Design review of the part built by this model. Coordinates are the model's own, in mm. A direction names the side the tool comes from. Give positions to 0.01 mm unless a question says otherwise; leave off trailing zeros. Order: outer loops, then holes, each group sorted by start corner. A loop starts at its lowest first (then second) coordinate and runs counter-clockwise, first axis right, second up. Notation, with made-up numbers: (-29, -17) -> (13, -17) arc R17 cw to (13, 16) -> close; hole circle Ø3 at (-19.75, -14). An arc over 180 degrees is marked (long way). One line per item, written item: value. Start each with the question number.
1) Wall thickness on line 1 along Z through (x, y) = (15.78, 1); line 2 along Z through (x, y) = (-15.78, 0.8); line 3 along X through (y, z) = (0.7, -8.3): over which ranges is each line inside the solid? List them lowest first. Write a range as from..to.
2) Consider section C-C (z = -8.9). State the section outline as (x, y) points (3 decimals), plus the area to 3 significant figures.
3) The part is to be moulded in two halves that separate along Z. For faces 1 (the face through (11.499, 4.958, -2.515)), 2 (the face through (6, 5, 9.4)), 3 (the face through (3.62, 12.1, -10)), say which applies: released by +Z, released by -Z, zero draft, split by the parting line, or undercut.
4) Tool access review of faces 4 (the face through (-12, 3, -4)), 5 (the face through (-20.276, 6.24, -0.694)), 6 (the face through (-0.115, 4.958, -2.499)), 7 (the face through (14.19, 0.66, 8.23)), 8 (the face through (6, 8.71, 3)): name each direction out of +Z, -Z, +X, -X, +Y, -Y from which nothing blocks a thin tool from reaching the whole face with its end or side.
5) Consider section D-D (y = 7.25). State the section outline as (x, z) points, plus the area to 3 significant figures.
6) For pin 1 (1 mm diameter, centred on x = 4, y = 6.5, fed in from +Z); pin 2 (2 mm diameter, centred on x = 4.5, y = 4, fed in from -Z); pin 3 (3 mm diameter, centred on x = -7.5, z = -4.5, fed in from +Y), all flat-tipped, find the tip position at first contact; note any pin that passes through.
7) Consider section A-A (y = 4). State the section outline as (x, z) points, plus the area to 3 significant figures.
8) Consider section B-B (x = 10). State the section outline as (y, z) points.
Autodesk Inventor part; units mm, degrees
ref_plane "YZ Plane" through (0, 0, 0) normal (1, 0, 0) x (0, 1, 0)
ref_plane "XZ Plane" through (0, 0, 0) normal (0, 1, 0) x (-1, 0, 0)
ref_plane "XY Plane" through (0, 0, 0) normal (0, 0, 1) x (1, 0, 0)
sketch "Sketch1" plane through (0, 0, 0) normal (0, 1, 0) x (-1, 0, 0)
  line L0 (21.5, -10.6) -> (-21.5, -10.6)
  line L1 (-21.5, -10.6) -> (-21.5, 10.6)
  line L2 (-21.5, 10.6) -> (21.5, 10.6)
  line L3 (21.5, 10.6) -> (21.5, -10.6)
  point P0 (0, 0)
  dimension "d0" = 43
  dimension "d1" = 21.2
  dimension "d2" = 10.6
  dimension "d3" = 21.5
extrude "Extrusion1" add sketch "Sketch1" along normal blind 1.31
sketch "Sketch2" plane through (0, 1.31, 0) normal (0, 1, 0) x (1, 0, 0)
  line L0 (-12, 10) -> (-1.85, 10)
  line L1 (-1.85, 10) -> (-1.85, -2.4)
  line L2 (-1.85, -2.4) -> (-12, -2.4)
  line L3 (-12, -2.4) -> (-12, 10)
  line L4 (-21.5, -10.6) -> (21.5, -10.6)
  line L5 (-21.5, 10.6) -> (-21.5, -10.6)
  point P0 (0, 0)
  dimension "d6" = 12.4
  dimension "d7" = 10.15
  dimension "d8" = 8.2
  dimension "d9" = 9.5
extrude "Extrusion2" add sketch "Sketch2" along normal blind 4
sketch "Sketch3" plane through (0, 1.31, 0) normal (0, 1, 0) x (1, 0, 0)
  line L0 (0.6, 2.8) -> (10.8, 2.8)
  line L1 (11.8, 1.8) -> (11.8, -8.4)
  line L2 (10.8, -9.4) -> (0.6, -9.4)
  line L3 (-0.4, -8.4) -> (-0.4, 1.8)
  line L4 (-21.5, -10.6) -> (21.5, -10.6)
  line L5 (21.5, -10.6) -> (21.5, 10.6)
  arc A0 (0.6, 2.8) -> (-0.4, 1.8) centre (0.6, 1.8) ccw
  arc A1 (11.8, 1.8) -> (10.8, 2.8) centre (10.8, 1.8) ccw
  arc A2 (10.8, -9.4) -> (11.8, -8.4) centre (10.8, -8.4) ccw
  arc A3 (-0.4, -8.4) -> (0.6, -9.4) centre (0.6, -8.4) ccw
  point P0 (0, 0)
  dimension "d12" = 12.2
  dimension "d13" = 12.2
  dimension "d14" = 1.2
  dimension "d15" = 9.7
  dimension "d16" = 1
extrude "Extrusion3" add sketch "Sketch3" along normal blind 7.4
sketch "Sketch4" plane through (0, 1.31, 0) normal (0, 1, 0) x (1, 0, 0)
  line L0 (2.66, 10.1) -> (12.13, 10.1)
  line L1 (12.13, 10.1) -> (12.13, 5.79)
  line L2 (12.13, 5.79) -> (2.66, 5.79)
  line L3 (2.66, 5.79) -> (2.66, 10.1)
  line L4 (21.5, -10.6) -> (21.5, 10.6)
  line L5 (21.5, 10.6) -> (-21.5, 10.6)
  point P0 (0, 0)
  dimension "d19" = 4.31
  dimension "d20" = 9.47
  dimension "d21" = 9.37
  dimension "d22" = 0.5
extrude "Extrusion4" add sketch "Sketch4" along normal blind 10
sketch "Sketch5" plane through (0, 11.31, 0) normal (0, 1, 0) x (1, 0, 0)
  circle A0 centre (3.86, 8.9) radius 1.125
  line L0 (12.13, 10.1) -> (2.66, 10.1)
  line L1 (2.66, 10.1) -> (2.66, 5.79)
  point P0 (0, 0)
  point P1 (2.66, 9.2358)
  point P2 (2.66, 8.7642)
  point P3 (4.0958, 10.1)
  point P4 (3.6242, 10.1)
  dimension "d25" = 2.25
  dimension "d26" = 1.2
  dimension "d27" = 1.2
extrude "Extrusion5" add sketch "Sketch5" along normal blind 1.61
sketch "Sketch6" plane through (0, 1.31, 0) normal (0, 1, 0) x (1, 0, 0)
  circle A0 centre (-16.28, 0.87) radius 4
  circle A1 centre (16.93, 1.23) radius 4
  line L0 (-21.5, -10.6) -> (21.5, -10.6)
  line L1 (21.5, -10.6) -> (21.5, 10.6)
  line L2 (-21.5, 10.6) -> (-21.5, -10.6)
  point P0 (0, 0)
  dimension "d30" = 8
  dimension "d31" = 8
  dimension "d32" = 11.83
  dimension "d33" = 4.57
  dimension "d34" = 5.22
  dimension "d35" = 11.47
extrude "Extrusion6" add sketch "Sketch6" along normal blind 10.5
fillet "Fillet1" radius 0.5 2 edges at (12.93, 11.81, -1.23) (-20.28, 11.81, -0.87)
sketch "Sketch7" plane through (0, 1.31, 0) normal (0, 1, 0) x (1, 0, 0)
  circle A0 centre (-15.78, 8.3) radius 1.59
  circle A1 centre (15.78, -8.3) radius 1.59
  line L0 (21.5, -10.6) -> (21.5, 10.6)
  line L1 (-21.5, -10.6) -> (21.5, -10.6)
  line L2 (21.5, 10.6) -> (-21.5, 10.6)
  line L3 (-21.5, 10.6) -> (-21.5, -10.6)
  point P0 (0, 0)
  dimension "d39" = 3.18
  dimension "d42" = 3.18
  dimension "d43" = 5.72
  dimension "d44" = 2.3
  dimension "d45" = 2.3
  dimension "d46" = 5.72
extrude "Extrusion7" cut sketch "Sketch7" against normal blind 3.18 contours A0 | A1
equation "\"d42\" = d39"
equation "\"d47\" = d39"
properties part number "Power Buck Converter"
Checked values:
1. line 1: z = -10.6..6.71, 9.89..10.6
1. line 2: z = -10.6..-9.89, -6.71..10.6
1. line 3: x = -21.5..-17.37, -14.19..21.5
2. outline: (-21.5, 0) -> (-17.252, 0) -> (-17.252, 1.31) -> (-21.5, 1.31) -> close; (-14.308, 0) -> (21.5, 0) -> (21.5, 1.31) -> (12.13, 1.31) -> (12.13, 11.31) -> (4.985, 11.31) -> (4.985, 12.92) -> (2.735, 12.92) -> (2.735, 11.31) -> (2.66, 11.31) -> (2.66, 1.31) -> (-1.85, 1.31) -> (-1.85, 5.31) -> (-12, 5.31) -> (-12, 1.31) -> (-14.308, 1.31) -> close
2. area: 191 mm^2
3. face 1: undercut
3. face 2: released by +Z
3. face 3: split by the parting line
4. face 4: +Z, -Z, +Y
4. face 5: +Y
4. face 6: -Z, +Y
4. face 7: +Y, -Y
4. face 8: +Z, +Y
5. outline: circle Ø8 at (-16.28, -0.87); (-0.4, -1.8) arc R1 ccw to (0.6, -2.8) -> (10.8, -2.8) arc R1 ccw to (11.8, -1.8) -> (11.8, 8.4) arc R1 ccw to (10.8, 9.4) -> (0.6, 9.4) arc R1 ccw to (-0.4, 8.4) -> close; (2.66, -10.1) -> (12.13, -10.1) -> (12.13, -5.79) -> (2.66, -5.79) -> close; circle Ø8 at (16.93, -1.23)
5. area: 289 mm^2
6. pin 1: stops at z = 9.4
6. pin 2: stops at z = -10.1
6. pin 3: stops at y = 5.31
7. outline: circle Ø8 at (-16.28, -0.87); (-12, -10) -> (-1.85, -10) -> (-1.85, 2.4) -> (-12, 2.4) -> close; (-0.4, -1.8) arc R1 ccw to (0.6, -2.8) -> (10.8, -2.8) arc R1 ccw to (11.8, -1.8) -> (11.8, 8.4) arc R1 ccw to (10.8, 9.4) -> (0.6, 9.4) arc R1 ccw to (-0.4, 8.4) -> close; (2.66, -10.1) -> (12.13, -10.1) -> (12.13, -5.79) -> (2.66, -5.79) -> close; circle Ø8 at (16.93, -1.23)
7. area: 415 mm^2
8. outline: (0, -10.6) -> (1.31, -10.6) -> (1.31, -10.1) -> (11.31, -10.1) -> (11.31, -5.79) -> (1.31, -5.79) -> (1.31, -2.8) -> (8.71, -2.8) -> (8.71, 9.4) -> (1.31, 9.4) -> (1.31, 10.6) -> (0, 10.6) -> close
